Part model, mm, in its own coordinate system. A direction names the side the tool comes from. Give positions to 0.01 mm unless a question says otherwise; leave off trailing zeros. Write each loop counter-clockwise with the first axis right and the second up, starting at its lowest first coordinate (ties: lowest second). Pieces come first, ordered by that corner, then holes.
```python
from build123d import *

# Parameters (mm, degrees)
SKETCH1_W           = 42
SKETCH1_H           = 24
BOSS_EXTRUDE1_DEPTH = 3
SKETCH2_W           = 4
SKETCH2_H           = 24
BOSS_EXTRUDE2_DEPTH = 24
SKETCH3_R           = 2.1
CUT_EXTRUDE1_DEPTH  = 52.351728306
SKETCH4_R           = 7.8
CUT_EXTRUDE2_DEPTH  = 1.6
CUT_EXTRUDE3_REACH  = 53.352
SKETCH5_R           = 1
CHAMFER1_SIZE       = 1.2
FILLET1_R           = 2.5
FILLET2_R           = 2.5
FILLET3_R           = 2.5
FILLET4_R           = 2.5
CUT_EXTRUDE4_REACH  = 38.249
SKETCH6_R           = 2.1
SKETCH7_R           = 4.7
CUT_EXTRUDE5_DEPTH  = 1.25
BOSS_EXTRUDE3_DEPTH = 1.6999
CUT_EXTRUDE6_REACH  = 53.352
BOSS_EXTRUDE4_DEPTH = 1.6999
SKETCH12_R          = 9.6
CUT_EXTRUDE7_DEPTH  = 1
CUT_EXTRUDE8_REACH  = 37.511
SKETCH13_R          = 1.1303
BOSS_EXTRUDE5_DEPTH = 0.75
CUT_EXTRUDE9_DEPTH  = 41.832517189
CUT_EXTRUDE10_DEPTH = 41.832517189
CUT_EXTRUDE11_DEPTH = 42.785164832
SKETCH19_R          = 2.875
CUT_EXTRUDE12_DEPTH = 1


with BuildPart() as part:
    # Sketch1 → Boss-Extrude1 (new body)
    with BuildSketch(Plane(origin=(0, 0, 0), x_dir=(1, 0, 0), z_dir=(0, 1, 0))):
        Rectangle(SKETCH1_W, SKETCH1_H)
    extrude(amount=BOSS_EXTRUDE1_DEPTH)

    # Sketch2 → Boss-Extrude2 (add)
    with BuildSketch(Plane(origin=(0, 3, 0), x_dir=(1, 0, 0), z_dir=(0, 1, 0))):
        with Locations((19, 0)):
            Rectangle(SKETCH2_W, SKETCH2_H)
        with Locations((-19, 0)):
            Rectangle(SKETCH2_W, SKETCH2_H)
    extrude(amount=BOSS_EXTRUDE2_DEPTH)

    # Sketch3 → Cut-Extrude1 (cut, through all)
    with BuildSketch(Plane(origin=(21, 0, 0), x_dir=(0, 0, -1), z_dir=(1, 0, 0))):
        with Locations((0, 17)):
            Circle(SKETCH3_R)
    extrude(amount=-CUT_EXTRUDE1_DEPTH, mode=Mode.SUBTRACT)

    # Sketch4 → Cut-Extrude2 (cut)
    with BuildSketch(Plane.ZY.offset(-17)):
        with Locations((0, 17)):
            Circle(SKETCH4_R)
    extrude(amount=-CUT_EXTRUDE2_DEPTH, mode=Mode.SUBTRACT)

    # Sketch5 → Cut-Extrude3 (cut, up to next)
    with BuildSketch(Plane(origin=(21, 0, 0), x_dir=(0, 0, -1), z_dir=(1, 0, 0)), mode=Mode.PRIVATE) as cut_extrude3_sk1:
        with Locations((-8, 25)):
            Circle(SKETCH5_R)
    cut_extrude3_tool1 = extrude(cut_extrude3_sk1.sketch, amount=-CUT_EXTRUDE3_REACH, mode=Mode.PRIVATE) & part.part
    # Sketch5 → Cut-Extrude3 (cut, up to next)
    with BuildSketch(Plane(origin=(21, 0, 0), x_dir=(0, 0, -1), z_dir=(1, 0, 0)), mode=Mode.PRIVATE) as cut_extrude3_sk2:
        with Locations((8, 25)):
            Circle(SKETCH5_R)
    cut_extrude3_tool2 = extrude(cut_extrude3_sk2.sketch, amount=-CUT_EXTRUDE3_REACH, mode=Mode.PRIVATE) & part.part
    # Sketch5 → Cut-Extrude3 (cut, up to next)
    with BuildSketch(Plane(origin=(21, 0, 0), x_dir=(0, 0, -1), z_dir=(1, 0, 0)), mode=Mode.PRIVATE) as cut_extrude3_sk3:
        with Locations((8, 9)):
            Circle(SKETCH5_R)
    cut_extrude3_tool3 = extrude(cut_extrude3_sk3.sketch, amount=-CUT_EXTRUDE3_REACH, mode=Mode.PRIVATE) & part.part
    # Sketch5 → Cut-Extrude3 (cut, up to next)
    with BuildSketch(Plane(origin=(21, 0, 0), x_dir=(0, 0, -1), z_dir=(1, 0, 0)), mode=Mode.PRIVATE) as cut_extrude3_sk4:
        with Locations((-8, 9)):
            Circle(SKETCH5_R)
    cut_extrude3_tool4 = extrude(cut_extrude3_sk4.sketch, amount=-CUT_EXTRUDE3_REACH, mode=Mode.PRIVATE) & part.part
    add(cut_extrude3_tool1.solids().sort_by_distance((21, 25, 8))[0], mode=Mode.SUBTRACT)
    add(cut_extrude3_tool2.solids().sort_by_distance((21, 25, -8))[0], mode=Mode.SUBTRACT)
    add(cut_extrude3_tool3.solids().sort_by_distance((21, 9, -8))[0], mode=Mode.SUBTRACT)
    add(cut_extrude3_tool4.solids().sort_by_distance((21, 9, 8))[0], mode=Mode.SUBTRACT)

    # Chamfer1
    # the kernel refuses this chamfer: 1.2 mm, written as the material it takes off along each edge
    with BuildSketch(Plane(origin=(21, 9, 8), x_dir=(0, 0, -1), z_dir=(0, -1, 0))) as chamfer1_piece_1:
        Polygon((1 + CHAMFER1_SIZE, 0), (1, -CHAMFER1_SIZE), (1, 0), align=None)
    revolve(axis=Axis((21, 9, 8), (1, 0, 0)), mode=Mode.SUBTRACT)
    with BuildSketch(Plane(origin=(21, 9, -8), x_dir=(0, 0, -1), z_dir=(0, -1, 0))) as chamfer1_piece_2:
        Polygon((1 + CHAMFER1_SIZE, 0), (1, -CHAMFER1_SIZE), (1, 0), align=None)
    revolve(axis=Axis((21, 9, -8), (1, 0, 0)), mode=Mode.SUBTRACT)
    with BuildSketch(Plane(origin=(21, 25, -8), x_dir=(0, 0, -1), z_dir=(0, -1, 0))) as chamfer1_piece_3:
        Polygon((1 + CHAMFER1_SIZE, 0), (1, -CHAMFER1_SIZE), (1, 0), align=None)
    revolve(axis=Axis((21, 25, -8), (1, 0, 0)), mode=Mode.SUBTRACT)
    with BuildSketch(Plane(origin=(21, 25, 8), x_dir=(0, 0, -1), z_dir=(0, -1, 0))) as chamfer1_piece_4:
        Polygon((1 + CHAMFER1_SIZE, 0), (1, -CHAMFER1_SIZE), (1, 0), align=None)
    revolve(axis=Axis((21, 25, 8), (1, 0, 0)), mode=Mode.SUBTRACT)

    # Fillet1
    fillet1_edges = [part.edges().sort_by_distance(p)[0] for p in [
        (19, 27, 12),
    ]]
    fillet(fillet1_edges, radius=FILLET1_R)

    # Fillet2
    fillet2_edges = [part.edges().sort_by_distance(p)[0] for p in [
        (19, 27, -12),
    ]]
    fillet(fillet2_edges, radius=FILLET2_R)

    # Fillet3
    fillet3_edges = [part.edges().sort_by_distance(p)[0] for p in [
        (-19, 27, -12),
    ]]
    fillet(fillet3_edges, radius=FILLET3_R)

    # Fillet4
    fillet4_edges = [part.edges().sort_by_distance(p)[0] for p in [
        (-19, 27, 12),
    ]]
    fillet(fillet4_edges, radius=FILLET4_R)

    # Sketch6 → Cut-Extrude4 (cut, up to next)
    with BuildSketch(Plane.XZ, mode=Mode.PRIVATE) as cut_extrude4_sk1:
        with Locations(Location((0, 0, 0), (0, 0, 270))):
            Circle(SKETCH6_R)
    cut_extrude4_tool1 = extrude(cut_extrude4_sk1.sketch, amount=-CUT_EXTRUDE4_REACH, mode=Mode.PRIVATE) & part.part
    add(cut_extrude4_tool1.solids().sort_by_distance((0, 0, 0))[0], mode=Mode.SUBTRACT)

    # Sketch7 → Cut-Extrude5 (cut)
    with BuildSketch(Plane(origin=(21, 0, 0), x_dir=(0, 0, -1), z_dir=(1, 0, 0))):
        with Locations((0, 17)):
            Circle(SKETCH7_R)
    cut_extrude5 = extrude(amount=-CUT_EXTRUDE5_DEPTH, mode=Mode.SUBTRACT)

    # Mirror1: Cut-Extrude5 across plane
    add(cut_extrude5.mirror(Plane(origin=(0, 0, 0), x_dir=(0, 0, 1), z_dir=(1, 0, 0))), mode=Mode.SUBTRACT)

    # Sketch9 → Boss-Extrude3 (add)
    with BuildSketch(Plane.XY.offset(12)):
        Polygon((-17, 3), (-17, 11), (-6, 3), align=None)
        Polygon((17, 11), (6, 3), (17, 3), align=None)
    extrude(amount=-BOSS_EXTRUDE3_DEPTH)

    # Sketch10 → Cut-Extrude6 (cut, up to next)
    with BuildSketch(Plane(origin=(21, 0, 0), x_dir=(0, 0, -1), z_dir=(1, 0, 0)), mode=Mode.PRIVATE) as cut_extrude6_sk1:
        with BuildLine():
            Line((2.1, 17), (2.1, 27))
            Line((2.1, 27), (-2.1, 27))
            Line((-2.1, 27), (-2.1, 17))
            ThreePointArc((-2.1, 17), (0, 14.9), (2.1, 17))
        make_face()
    cut_extrude6_tool1 = extrude(cut_extrude6_sk1.sketch, amount=-CUT_EXTRUDE6_REACH, mode=Mode.PRIVATE) & part.part
    add(cut_extrude6_tool1.solids().sort_by_distance((21, 21.165903, 0))[0], mode=Mode.SUBTRACT)

    # Sketch11 → Boss-Extrude4 (add)
    with BuildSketch(Plane(origin=(0, 0, -12), x_dir=(-1, 0, 0), z_dir=(0, 0, -1))):
        Polygon((-17, 3), (-17, 11), (-6, 3), align=None)
        Polygon((17, 11), (6, 3), (17, 3), align=None)
    extrude(amount=-BOSS_EXTRUDE4_DEPTH)

    # Sketch12 → Cut-Extrude7 (cut)
    with BuildSketch(Plane.XZ):
        with Locations(Location((0, 0, 0), (0, 0, 270))):
            Circle(SKETCH12_R)
    extrude(amount=-CUT_EXTRUDE7_DEPTH, mode=Mode.SUBTRACT)

    # Sketch13 → Cut-Extrude8 (cut, up to next)
    with BuildSketch(Plane.XZ.offset(-1), mode=Mode.PRIVATE) as cut_extrude8_sk1:
        with Locations(Location((-4.49015, 4.49015, 0), (0, 0, 270))):
            Circle(SKETCH13_R)
    cut_extrude8_tool1 = extrude(cut_extrude8_sk1.sketch, amount=-CUT_EXTRUDE8_REACH, mode=Mode.PRIVATE) & part.part
    # Sketch13 → Cut-Extrude8 (cut, up to next)
    with BuildSketch(Plane.XZ.offset(-1), mode=Mode.PRIVATE) as cut_extrude8_sk2:
        with Locations(Location((4.49015, 4.49015, 0), (0, 0, 270))):
            Circle(SKETCH13_R)
    cut_extrude8_tool2 = extrude(cut_extrude8_sk2.sketch, amount=-CUT_EXTRUDE8_REACH, mode=Mode.PRIVATE) & part.part
    # Sketch13 → Cut-Extrude8 (cut, up to next)
    with BuildSketch(Plane.XZ.offset(-1), mode=Mode.PRIVATE) as cut_extrude8_sk3:
        with Locations(Location((4.49015, -4.49015, 0), (0, 0, 270))):
            Circle(SKETCH13_R)
    cut_extrude8_tool3 = extrude(cut_extrude8_sk3.sketch, amount=-CUT_EXTRUDE8_REACH, mode=Mode.PRIVATE) & part.part
    # Sketch13 → Cut-Extrude8 (cut, up to next)
    with BuildSketch(Plane.XZ.offset(-1), mode=Mode.PRIVATE) as cut_extrude8_sk4:
        with Locations(Location((-4.49015, -4.49015, 0), (0, 0, 270))):
            Circle(SKETCH13_R)
    cut_extrude8_tool4 = extrude(cut_extrude8_sk4.sketch, amount=-CUT_EXTRUDE8_REACH, mode=Mode.PRIVATE) & part.part
    add(cut_extrude8_tool1.solids().sort_by_distance((-4.49015, 1, 4.49015))[0], mode=Mode.SUBTRACT)
    add(cut_extrude8_tool2.solids().sort_by_distance((4.49015, 1, 4.49015))[0], mode=Mode.SUBTRACT)
    add(cut_extrude8_tool3.solids().sort_by_distance((4.49015, 1, -4.49015))[0], mode=Mode.SUBTRACT)
    add(cut_extrude8_tool4.solids().sort_by_distance((-4.49015, 1, -4.49015))[0], mode=Mode.SUBTRACT)

    # Sketch14 → Boss-Extrude5 (add)
    with BuildSketch(Plane(origin=(0, 3, 0), x_dir=(1, 0, 0), z_dir=(0, 1, 0))):
        Polygon((-6, 10.3001), (-11.5, 0), (-6, -10.3001), (-7.01769667, -10.3001), (-12.008848335, -0.952943406), (-17, -10.3001), (-17, -8.389390136), (-12.518984365, 0.002411526), (-17, 8.394213188), (-17, 10.3001), (-12.01013603, 0.955354932), (-7.020272061, 10.3001), align=None)
        Polygon((-9.738422165, -10.3001), (-12.008848335, -6.048169711), (-14.279274505, -10.3001), (-15.296971174, -10.3001), (-14.882917623, -9.519860041), (-12.01013603, -4.139871373), (-8.720725495, -10.3001), align=None)
        Polygon((-8.720725495, 10.3001), (-9.740997556, 10.3001), (-12.01013603, 6.050581237), (-14.279274505, 10.3001), (-15.296971174, 10.3001), (-12.008848335, 4.142282899), align=None)
        Polygon((14.882917623, -9.519860041), (12.01013603, -4.139871373), (8.720725495, -10.3001), (9.738422165, -10.3001), (12.008848335, -6.048169711), (14.279274505, -10.3001), (15.296971174, -10.3001), align=None)
        Polygon((12.01013603, 6.050581237), (9.740997556, 10.3001), (8.720725495, 10.3001), (12.008848335, 4.142282899), (15.296971174, 10.3001), (14.279274505, 10.3001), align=None)
        Polygon((12.008848335, -0.952943406), (17, -10.3001), (17, -8.389390136), (12.518984365, 0.002411526), (17, 8.394213188), (17, 10.3001), (12.01013603, 0.955354932), (7.020272061, 10.3001), (6, 10.3001), (11.5, 0), (6, -10.3001), (7.01769667, -10.3001), align=None)
    extrude(amount=BOSS_EXTRUDE5_DEPTH)

    # Sketch16 → Cut-Extrude9 (cut, through all)
    with BuildSketch(Plane.XY.offset(10.3001)):
        Polygon((-7.01769667, 3.740143032), (-6, 3), (-6, 3.75), (-7.01769667, 3.75), align=None)
    extrude(amount=-CUT_EXTRUDE9_DEPTH, mode=Mode.SUBTRACT)

    # Sketch17 → Cut-Extrude10 (cut, through all)
    with BuildSketch(Plane.XY.offset(10.3001)):
        Polygon((6, 3), (7.01769667, 3.740143032), (7.01769667, 3.75), (6, 3.75), align=None)
    extrude(amount=-CUT_EXTRUDE10_DEPTH, mode=Mode.SUBTRACT)

    # Sketch18 → Cut-Extrude11 (cut, through all)
    with BuildSketch(Plane(origin=(0, 0, -12), x_dir=(-1, 0, 0), z_dir=(0, 0, -1))):
        Polygon((15.296971174, 3.75), (17, 3.75), (17, 8.527005362), (10.431617627, 3.75), (14.279274505, 3.75), align=None)
        Polygon((-10.431617627, 3.75), (-17, 8.527005362), (-17, 3.75), (-15.296971174, 3.75), (-14.279274505, 3.75), align=None)
    extrude(amount=-CUT_EXTRUDE11_DEPTH, mode=Mode.SUBTRACT)

    # Sketch19 → Cut-Extrude12 (cut)
    with BuildSketch(Plane(origin=(0, 3, 0), x_dir=(1, 0, 0), z_dir=(0, 1, 0))):
        with Locations(Location((-4.49015, -4.49015, 0), (0, 0, 270))):
            Circle(SKETCH19_R)
        with Locations(Location((4.49015, -4.49015, 0), (0, 0, 270))):
            Circle(SKETCH19_R)
        with Locations(Location((-4.49015, 4.49015, 0), (0, 0, 270))):
            Circle(SKETCH19_R)
        with Locations(Location((4.49015, 4.49015, 0), (0, 0, 270))):
            Circle(SKETCH19_R)
    extrude(amount=-CUT_EXTRUDE12_DEPTH, mode=Mode.SUBTRACT)


solid = part.part
```
1) Pin check, flat tips, straight feed: pin 1 Ø3.5 at (x, z) = (13, 7.5) entering from +Y; pin 2 Ø3.5 at (x, z) = (4.49, 4.49) entering from -Y; pin 3 Ø5 at (y, z) = (16.5, -2) entering from +X. Stop position of each tip, or through.
Answers follow:
pin 1: stops at y = 3.75
pin 2: stops at y = 1
pin 3: stops at x = 19.75
2) Wall check: L1, parallel to Y at x = 18, z = 8; L2, parallel to X at y = 18, z = -9; L3, parallel to X at y = 15.75, z = 5. Give the ranges that are in metal, low to high.
Answers follow:
L1: y = 0 to 8, 10 to 24, 26 to 27
L2: x = -21 to -17, 17 to 21
L3: x = -21 to -17, 18.6 to 21
3) Saw through at A-A, the plane x = 0. Write the cut outline in (y, z).
Answers follow:
outline: (0, -12) - (3, -12) - (3, -2.1) - (1, -2.1) - (1, -9.6) - (0, -9.6) - close; (0, 9.6) - (1, 9.6) - (1, 2.1) - (3, 2.1) - (3, 12) - (0, 12) - close
4) 3-axis set-ups, long thin cutter, end or side, ignore diameter. For faces 4 (the face through (14, 3.75, -9)), 5 (the face through (-19, 27, 0)), 6 (the face through (-4, 2, -3)): which of +Z, -Z, +X, -X, +Y, -Y reach the whole face in a straight line?
Answers follow:
face 4: none
face 5: +Z, -Z, +X, -X, +Y
face 6: +Y
5) Saw through at C-C, the plane y = 25. Write the cut outline in (x, z).
Answers follow:
outline: (-21, -11.95) - (-17, -11.95) - (-17, 11.95) - (-21, 11.95) - close; (17, -11.95) - (21, -11.95) - (21, -10.2) - (19.8, -9) - (17, -9) - close; (17, -7) - (19.8, -7) - (21, -5.8) - (21, -2.1) - (17, -2.1) - close; (17, 2.1) - (21, 2.1) - (21, 5.8) - (19.8, 7) - (17, 7) - close; (17, 9) - (19.8, 9) - (21, 10.2) - (21, 11.95) - (17, 11.95) - close
6) Two-plate mould, pull along Y, no slides. Class faces 1 (the face through (-18.36, 18.77, -1.13)), 2 (the face through (-10, 0, 0)), 3 (the face through (-14.73, 3.37, -4.14)): +Y half, -Y half, draft (parallel to the pull), parting line (faces both ways), or undercut.
Answers follow:
face 1: undercut
face 2: -Y half
face 3: draft
7) Saw through at B-B, the plane y = 11.75. Write the cut outline in (x, z), then the cut area to 3 significant figures.
Answers follow:
outline: (-21, -12) - (-17, -12) - (-17, 12) - (-21, 12) - close; (17, -12) - (21, -12) - (21, 12) - (17, 12) - (17, 5.77) - (18.6, 5.77) - (18.6, -5.77) - (17, -5.77) - close
area: 174 mm2
